Verification items for the finished model (mm, model axes). Face numbers are marked on the shaded views. A direction names the side the tool comes from. Give positions to 0.01 mm unless a question says otherwise; leave off trailing zeros. Order: outer loops, then holes, each group sorted by start corner. A loop starts at its lowest first (then second) coordinate and runs counter-clockwise, first axis right, second up.
from build123d import *

# Parameters (mm, degrees)
BOSS_EXTRUDE1_DEPTH = 38.1
SKETCH2_R           = 6.35
BOSS_EXTRUDE2_DEPTH = 19.05
SKETCH3_R           = 2.2479
CUT_EXTRUDE1_DEPTH  = 42.275


with BuildPart() as part:
    # Sketch1 → Boss-Extrude1 (new body)
    with BuildSketch(Plane(origin=(0, 0, 0), x_dir=(0, 0, -1), z_dir=(1, 0, 0))):
        Polygon((-3.175, 0), (3.175, 0), (3.175, 19.05), (25.4, 19.05), (25.4, 25.4), (-25.4, 25.4), (-25.4, 19.05), (-3.175, 19.05), align=None)
    extrude(amount=BOSS_EXTRUDE1_DEPTH)

    # Sketch2 → Boss-Extrude2 (add)
    with BuildSketch(Plane.ZY):
        with BuildLine():
            ThreePointArc((-7.490824128, -5.312340931), (0, -15.875), (7.490824128, -5.312340931))
            Line((7.490824128, -5.312340931), (3.532340698, 5.983090093))
            ThreePointArc((3.532340698, 5.983090093), (3.264972581, 7.018061624), (3.175, 8.083217348))
            Line((3.175, 8.083217348), (3.175, 7.002752616))
            Line((3.175, 7.002752616), (3.175, 0))
            Line((3.175, 0), (-3.175, 0))
            Line((-3.175, 0), (-3.175, 7.002752616))
            Line((-3.175, 7.002752616), (-3.175, 8.083217348))
            ThreePointArc((-3.175, 8.083217348), (-3.264972581, 7.018061624), (-3.532340698, 5.983090093))
            Line((-3.532340698, 5.983090093), (-7.490824128, -5.312340931))
        make_face()
        with Locations((0, -7.9375)):
            Circle(SKETCH2_R, mode=Mode.SUBTRACT)
    extrude(amount=-BOSS_EXTRUDE2_DEPTH)

    # Sketch3 → Cut-Extrude1 (cut, through all)
    with BuildSketch(Plane(origin=(0, 25.4, 0), x_dir=(1, 0, 0), z_dir=(0, 1, 0))):
        with Locations((5.4229, 18.169466667)):
            Circle(SKETCH3_R)
        with Locations((32.6771, 18.169466667)):
            Circle(SKETCH3_R)
        with Locations((32.6771, -18.169466667)):
            Circle(SKETCH3_R)
        with Locations((5.4229, -18.169466667)):
            Circle(SKETCH3_R)
    extrude(amount=-CUT_EXTRUDE1_DEPTH, mode=Mode.SUBTRACT)


solid = part.part
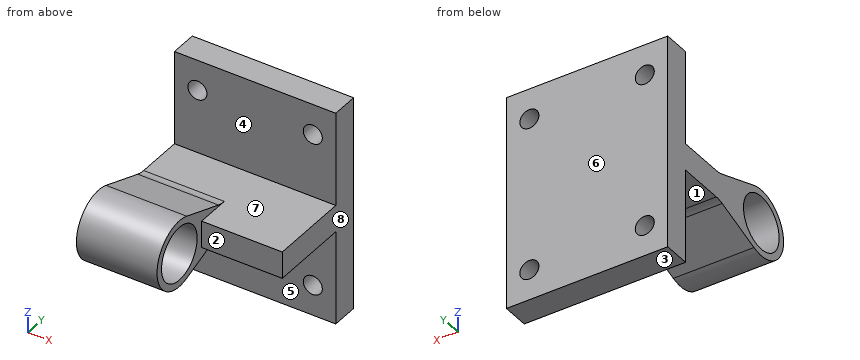
(1) Go/stop test with flat-tipped pins: pin 1 (6 mm diameter, centred on x = 32.68, z = 18.17, fed in from -Y); pin 2 (3 mm diameter, centred on x = 28, z = 0, fed in from -Y); pin 3 (4 mm diameter, centred on x = 25.5, y = 7, fed in from -Z) (3 decimals); pin 4 (17.5 mm diameter, centred on y = -6, z = 2, fed in from +X). Record where each tip stops, or that it passes through.
Solved:
pin 1: stops at y = 19.05
pin 2: stops at y = 0
pin 3: stops at z = -3.175
pin 4: stops at x = 38.1
(2) Scan lines: line 1 (X direction, y = 20, z = 17); line 2 (X direction, y = 23, z = 16.5); line 3 (Y direction, x = 29, z = 10.5). Record each from-to range of solid material in increasing order.
Solved:
line 1: x = 0 to 3.5, 7.34 to 30.76, 34.6 to 38.1
line 2: x = 0 to 3.92, 6.93 to 31.17, 34.18 to 38.1
line 3: y = 19.05 to 25.4
(3) Set-up check for the marked faces 4, 5, 6, 7 and 8: record each of +Z, -Z, +X, -X, +Y, -Y from which the full face is reachable in a straight line by a thin tool's end or side.
Solved:
face 4: +Z, +X, -X
face 5: -Z, +X, -X
face 6: +Z, -Z, +X, -X, +Y
face 7: +Z, +X
face 8: +Z, -Z, +X, +Y, -Y
(4) Section check C-C, the plane y = -11. Enter the section's corners in (x, z), then the cut area to 3 significant figures.
Solved:
outline: (0, -7.32) - (19.05, -7.32) - (19.05, -5.56) - (0, -5.56) - close; (0, 5.56) - (19.05, 5.56) - (19.05, 7.32) - (0, 7.32) - close
area: 67.1 mm2
(5) Section check B-B, the plane x = 29.5. Enter the section's corners in (y, z) (3 decimals).
Solved:
outline: (0, -3.175) - (19.05, -3.175) - (19.05, -25.4) - (25.4, -25.4) - (25.4, 25.4) - (19.05, 25.4) - (19.05, 3.175) - (0, 3.175) - close
(6) Release check for a two-part mould opening along Y. For the marked faces 1, 2 and 3 record: pulls with the +Y half, pulls with the -Y half, needs draft (parallel to the pull), parting line crosses it, or undercut.
Solved:
face 1: undercut
face 2: pulls with the -Y half
face 3: needs draft
